```python
from build123d import *

# Parameters (mm, degrees)
F0_W     = 100
F0_H     = 50
F1_DEPTH = 25
F2_R     = 10
F3_DEPTH = 25


# Not quite as in the source:
# - a pattern or mirror of a feature is missing from the dataset's text; its kind, count and spacing are read off the source's solid


with BuildPart() as f1:
    # F0 (on Top) → F1 (new body)
    with BuildSketch(Plane.XY):
        with Locations((0, 25)):
            Rectangle(F0_W, F0_H)
    extrude(amount=F1_DEPTH)

    # F2 (on face) → F3 (join, through all)
    with BuildSketch(Plane.XY.offset(25)):
        with Locations((-50, 25)):
            Circle(F2_R)
    f3 = extrude(amount=-F3_DEPTH)

    # F3_copies: F3 across plane
    add(f3.mirror(Plane(origin=(0, 0, 0), x_dir=(0, 0, 1), z_dir=(1, 0, 0))))


solid = f1.part
```
Work out the finished part from the listing and answer in its coordinate system (mm). A direction names the side the tool comes from. Give positions to 0.01 mm unless a question says otherwise; leave off trailing zeros. Loops run counter-clockwise (first coordinate to the right, second up) from the corner with the lowest first, then second, coordinate; pieces in that order, holes last. Notation, with made-up numbers: (67.25, -39) -> (101.25, -39) arc R14 cw to (101.25, -13) -> close; hole circle Ø6 at (28.25, -19.75). An arc over 180 degrees is marked (long way). One line per question, with ' | ' between items. Start each with the question number.
1) Section B-B, the plane y = 37.5 is taken. Determine the outline of the cut face in (x, z).
2) Each of these flat-tipped pins is pushed along its axis until it touches: pin 1 (5 mm diameter, centred on y = 6.5, z = 19, fed in from +X); pin 2 (1.5 mm diameter, centred on x = -17.5, y = 14, fed in from -Z); pin 3 (8 mm diameter, centred on y = 30.5, z = 19, fed in from +X); pin 4 (7.5 mm diameter, centred on y = 7.5, z = 15, fed in from -X). Where does it stop, or does it pass through?
3) Section A-A, the plane z = 20.75 is taken. Determine the outline of the cut face in (x, y), then the cut area to 3 significant figures.
4) Straight lines are drawn through the part: L1, parallel to X at y = 42.5, z = 3.5; L2, parallel to Y at x = 52.5, z = 5.25; L3, parallel to X at y = 19, z = 9.75. For each, find the intervals that lie inside material, in ascending order.
5) For faces 1 (the face through (50, 7, 12)), 2 (the face through (-50, 42, 12)), 3 (the face through (-50, 7, 12)), 4 (the face through (50, 42, 12)), 5 (the face through (-1, 0, 12)), determine the directions among +Z, -Z, +X, -X, +Y, -Y from which every point of the face is accessible in a straight line to the end or side of a thin tool.
Resolved:
1) outline: (-50, 0) -> (50, 0) -> (50, 25) -> (-50, 25) -> close
2) pin 1: x = 50 | pin 2: z = 0 | pin 3: x = 59.89 | pin 4: x = -50
3) outline: (-50, 0) -> (50, 0) -> (50, 15) arc R10 ccw to (50, 35) -> (50, 50) -> (-50, 50) -> (-50, 35) arc R10 ccw to (-50, 15) -> close | area: 5,310 mm2
4) L1: -50 to 50 | L2: 15.32 to 34.68 | L3: -58 to 58
5) face 1: +Z, -Z, +X, -Y | face 2: +Z, -Z, -X, +Y | face 3: +Z, -Z, -X, -Y | face 4: +Z, -Z, +X, +Y | face 5: +Z, -Z, +X, -X, -Y
